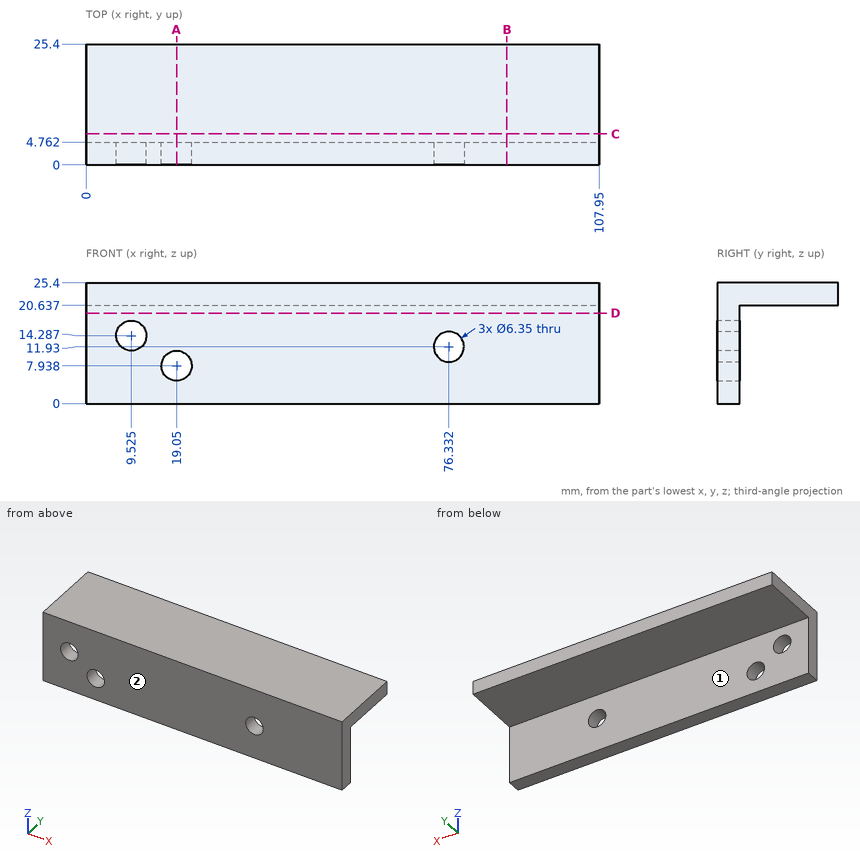
Input: dimensioned drawing with shaded views. Units: mm. Origin: part minimum x, y, z. A direction names the side the tool comes from. Coordinates: 2 decimals unless noted, no trailing zeros. Write each loop counter-clockwise with the first axis right and the second up, starting at its lowest first coordinate (ties: lowest second). Pieces come first, ordered by that corner, then holes. Notation, with made-up numbers: M 30,-33.5 L 66,-33.5 A25 ccw 66,-20.5 Z; hole C 24,38.25 d7. An arc over 180 degrees is marked long. Use a Markdown table: item, result.
1) Section C-C, the plane y = 6.5. Output: boundary loops of the cut face in (x, z), then the cut area to 3 significant figures.
Conclusion:
| item | result |
|---|---|
| outline | M 0,20.64 L 107.95,20.64 L 107.95,25.4 L 0,25.4 Z |
| area | 514 mm^2 |
2) Section B-B, the plane x = 88.5. Output: boundary loops of the cut face in (y, z), then the cut area to 3 significant figures.
Conclusion:
| item | result |
|---|---|
| outline | M 0,0 L 4.76,0 L 4.76,20.64 L 25.4,20.64 L 25.4,25.4 L 0,25.4 Z |
| area | 219 mm^2 |
3) Section A-A, the plane x = 19.05. Output: boundary loops of the cut face in (y, z).
Conclusion:
| item | result |
|---|---|
| outline | M 0,0 L 4.76,0 L 4.76,4.76 L 0,4.76 Z; M 0,11.11 L 4.76,11.11 L 4.76,20.64 L 25.4,20.64 L 25.4,25.4 L 0,25.4 Z |
4) Ray query, L1, parallel to Y at x = 78, z = 4.75; L2, parallel to Z at x = 35.5, y = 5; L3, parallel to Z at x = 19.5, y = 2.25 (1 decimal). Return the intervals inside material, ascending.
Conclusion:
| item | result |
|---|---|
| L1 | y = 0 to 4.76 |
| L2 | z = 20.64 to 25.4 |
| L3 | z = 0 to 4.8, 11.1 to 25.4 |
5) Reachability of the marked faces 1 and 2 from +Z, -Z, +X, -X, +Y, -Y: full face, straight path, thin tool, end or side. Return the list, or none.
Conclusion:
| item | result |
|---|---|
| face 1 | -Z, +X, -X, +Y |
| face 2 | +Z, -Z, +X, -X, -Y |
6) First-contact query: pin 1 Ø5.5 at (x, z) = (9.52, 14.29) entering from +Y; pin 2 Ø6 at (x, y) = (70.5, 8.5) entering from -Z; pin 3 Ø10.5 at (x, z) = (40, 6) entering from +Y. Flat tips, straight axial feed; report the tip coordinate or a pass-through.
Conclusion:
| item | result |
|---|---|
| pin 1 | passes through |
| pin 2 | stops at z = 20.64 |
| pin 3 | stops at y = 4.76 |
7) Section D-D, the plane z = 19. Output: boundary loops of the cut face in (x, y).
Conclusion:
| item | result |
|---|---|
| outline | M 0,0 L 107.95,0 L 107.95,4.76 L 0,4.76 Z |
